Geometry: see drawing. Coordinates: mm, zero at the bounding-box minimum. Round coordinates to 2 decimals unless told otherwise and drop trailing zeros. Order: outer loops, then holes, each group sorted by start corner. A loop starts at its lowest first (then second) coordinate and runs counter-clockwise, first axis right, second up. Notation, with made-up numbers: (86.25, 54) -> (114.25, 54) arc R30 cw to (114.25, 79) -> close; hole circle Ø3 at (29.25, -35.75). An arc over 180 degrees is marked (long way). Write item = value, one per line. Start each with the question number.
(1) Cut plane D-D on y = 6.25. Return the cut outline in (x, z).
(2) Cut plane C-C on y = 4. Return the cut outline in (x, z), then the cut area to 3 significant figures.
(3) Draft query along Y for the marked faces 1, 2 and 3. Return one class per face: released by +Y, released by -Y, zero draft, split by the parting line, or undercut.
(4) Cut plane A-A on z = 3.25. Return the cut outline in (x, y).
(5) Cut plane B-B on x = 18.5. Return the cut outline in (y, z).
(6) Ray query, line 1 (X direction, y = 2.75, z = 1.75); line 2 (X direction, y = 3.25, z = 7.75); line 3 (Y direction, x = 18.5, z = 2.75). Return the intervals inside material, ascending.
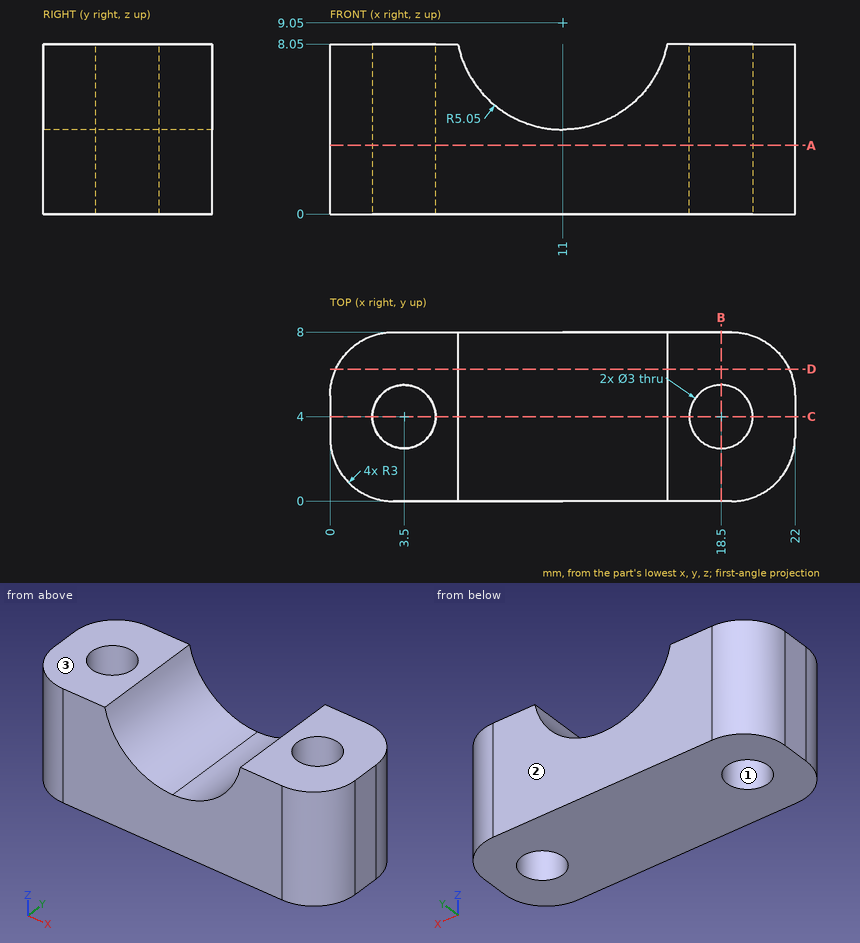
Evaluation:
q1.outline = (0.27, 0) -> (21.73, 0) -> (21.73, 8.05) -> (15.95, 8.05) arc R5.05 cw to (6.05, 8.05) -> (0.27, 8.05) -> close
q2.outline = (0, 0) -> (2, 0) -> (2, 8.05) -> (0, 8.05) -> close; (5, 0) -> (17, 0) -> (17, 8.05) -> (15.95, 8.05) arc R5.05 cw to (6.05, 8.05) -> (5, 8.05) -> close; (20, 0) -> (22, 0) -> (22, 8.05) -> (20, 8.05) -> close
q2.area = 98.8 mm^2
q3.face_1 = undercut
q3.face_2 = released by +Y
q3.face_3 = zero draft
q4.outline = (0, 3) arc R3 ccw to (3, 0) -> (19, 0) arc R3 ccw to (22, 3) -> (22, 5) arc R3 ccw to (19, 8) -> (3, 8) arc R3 ccw to (0, 5) -> close; hole circle Ø3 at (3.5, 4); hole circle Ø3 at (18.5, 4)
q5.outline = (0, 0) -> (2.5, 0) -> (2.5, 8.05) -> (0, 8.05) -> close; (5.5, 0) -> (8, 0) -> (8, 8.05) -> (5.5, 8.05) -> close
q6.line_1 = 0.01 to 2.67, 4.33 to 17.67, 19.33 to 21.99
q6.line_2 = 0 to 2.2, 4.8 to 6.12, 15.88 to 17.2, 19.8 to 22
q6.line_3 = 0 to 2.5, 5.5 to 8
